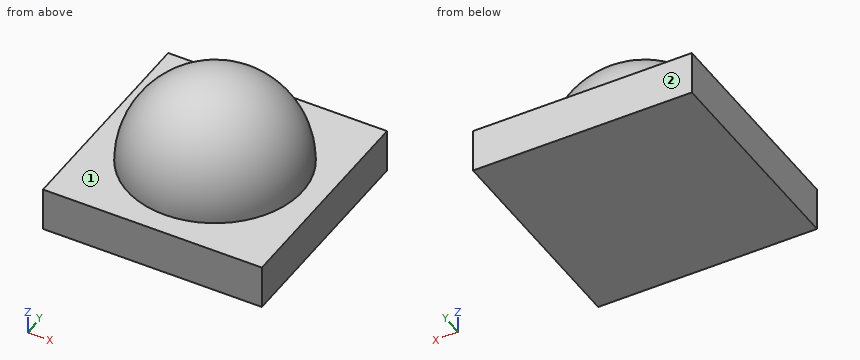
```python
from build123d import *

# Parameters (mm, degrees)
F0_W     = 25
F0_H     = 25
F1_DEPTH = 5
F3_ANGLE = 180


with BuildPart() as f1:
    # F0 (on Top) → F1 (new body)
    with BuildSketch(Plane.XY):
        Rectangle(F0_W, F0_H)
    extrude(amount=F1_DEPTH)

    # F2 (on face) → F3 (revolve)
    with BuildSketch(Plane.XY.offset(5)):
        with BuildLine():
            Line((0, -10), (0, 10))
            ThreePointArc((0, 10), (-10, 0), (0, -10))
        make_face()
    revolve(axis=Axis((0, 0, 5), (0, 1, 0)), revolution_arc=F3_ANGLE)


solid = f1.part
```
Design review of the part built by this model. Coordinates are the model's own, in mm. Face numbers are marked on the shaded views. A direction names the side the tool comes from. Round coordinates to 2 decimals unless told otherwise and drop trailing zeros. Order: outer loops, then holes, each group sorted by start corner. A loop starts at its lowest first (then second) coordinate and runs counter-clockwise, first axis right, second up. Notation, with made-up numbers: M 32.5,78.5 L 84.5,78.5 A36 ccw 84.5,115.5 Z; hole C 83,55 d10. An arc over 180 degrees is marked long. Put each result on its own line as item: value.
Q1. To check wall thickness, follow line 1 (Z direction, x = 9.75, y = 4); line 2 (X direction, y = -1.5, z = 7.5); line 3 (Y direction, x = 0.75, z = 6). State the ranges of each line that lie inside material, in increasing order.
Reported:
line 1: 0 to 5
line 2: -9.57 to 9.57
line 3: -9.92 to 9.92
Q2. Consider section D-D (y = -8.5). State the section outline as (x, z) points.
Reported:
outline: M -12.5,0 L 12.5,0 L 12.5,5 L 5.27,5 A5.27 ccw -5.27,5 L -12.5,5 Z
Q3. Insertion check: pin 1 Ø8 at (x, y) = (10, -6.5) entering from +Z; pin 2 Ø10 at (x, y) = (-6, 6.5) entering from +Z; pin 3 Ø1 at (y, z) = (2.5, 6.5) entering from -X. Each pin has a flat end and moves straight along its axis. Give the tip position at first contact, or say it passes through.
Reported:
pin 1: z = 11.1
pin 2: z = 14.23
pin 3: x = -9.7
Q4. Consider section B-B (x = 10.5). State the section outline as (y, z) points, and give its area (3 significant figures).
Reported:
outline: M -12.5,0 L 12.5,0 L 12.5,5 L -12.5,5 Z
area: 125 mm²
Q5. Consider section C-C (z = 6.75). State the section outline as (x, y) points, and give its area (3 significant figures).
Reported:
outline: C 0,0 d19.69
area: 305 mm²
Q6. Machinability: for the marked faces 1 and 2, which of the approach directions +Z, -Z, +X, -X, +Y, -Y give a long, thin tool a straight path to every point of the face, cutting with its end or side? Answer none if there is none.
Reported:
face 1: +Z
face 2: +Z, -Z, +X, -X, +Y
Q7. Consider section A-A (y = -2). State the section outline as (x, z) points, and give its area (3 significant figures).
Reported:
outline: M -12.5,0 L 12.5,0 L 12.5,5 L 9.8,5 A9.8 ccw -9.8,5 L -12.5,5 Z
area: 276 mm²
